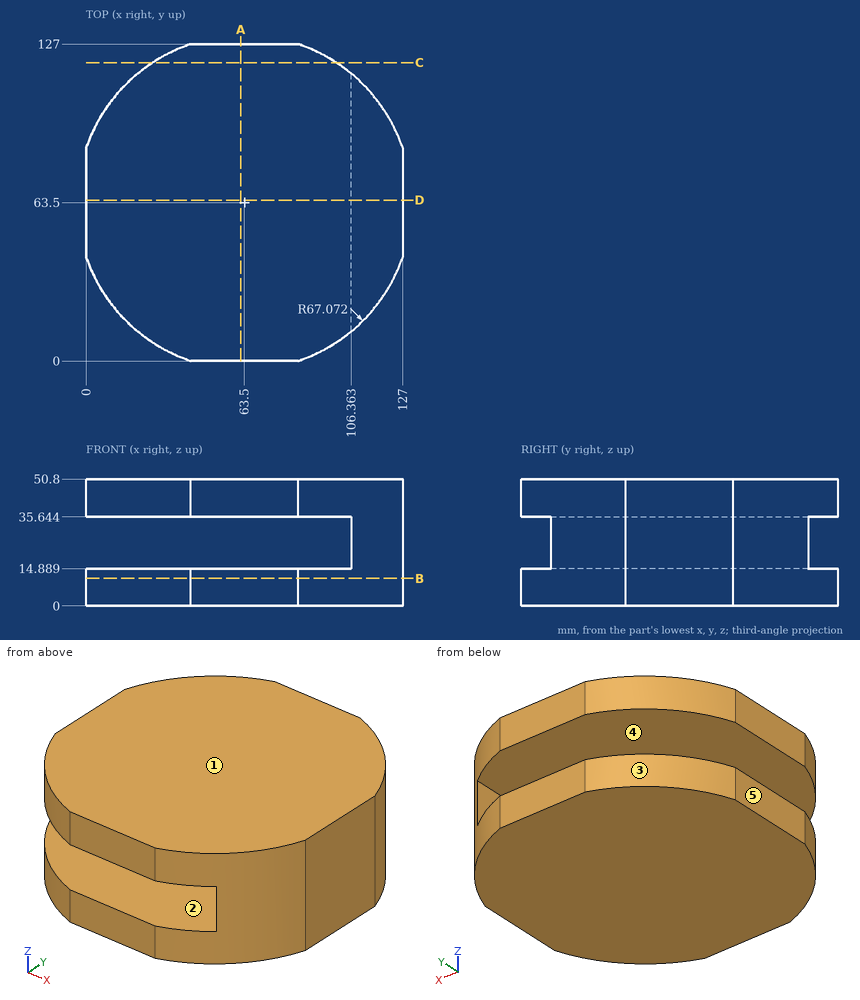
Study the drawing (mm; zero at the part's minimum x, y, z) and answer. A direction names the side the tool comes from. Give positions to 0.01 mm unless a question says otherwise; leave off trailing zeros. Order: outer loops, then holes, each group sorted by start corner. A loop starts at its lowest first (then second) coordinate and runs counter-clockwise, first axis right, second up. Notation, with made-up numbers: (57, -24.75) -> (80, -24.75) arc R20 ccw to (80, 14.25) -> close; hole circle Ø11 at (-10.75, 29). An arc over 180 degrees is marked (long way). Put each result on its own line as item: value.
Item 1: A cutting plane is placed at B-B on z = 11. Give the vertices of the cut face in (x, y) (1 decimal), plus the area to 3 significant figures.
Established:
outline: (0, 41.9) arc R67.1 ccw to (41.9, 0) -> (85.1, 0) arc R67.1 ccw to (127, 41.9) -> (127, 85.1) arc R67.1 ccw to (85.1, 127) -> (41.9, 127) arc R67.1 ccw to (0, 85.1) -> close
area: 13,700 mm^2
Item 2: For the marked faces 4 and 5, determine the directions among +Z, -Z, +X, -X, +Y, -Y from which every point of the face is accessible in a straight line to the end or side of a thin tool.
Established:
face 4: -X, +Y, -Y
face 5: +Z, -Z, -X, +Y, -Y
Item 3: Given P1, Ø1, axis at y = 95, z = 36, coming from the +X side; P2, Ø1.5, axis at x = 37.5, z = 34.5, coming from the -Y side; P3, Ø2, axis at y = 28, z = 29.5, coming from the -X side; P4, Ø10, axis at y = 20.5, z = 12.5, coming from the +X side, each flat-ended and moving along its own axis, determine where each tip first touches the part or whether it passes through.
Established:
P1: stops at x = 122.98
P2: passes through
P3: stops at x = 106.36
P4: stops at x = 118.77
Item 4: A cutting plane is placed at A-A on x = 62. Give the vertices of the cut face in (y, z).
Established:
outline: (0, 0) -> (127, 0) -> (127, 14.89) -> (0, 14.89) -> close; (0, 35.64) -> (127, 35.64) -> (127, 50.8) -> (0, 50.8) -> close
Item 5: For a pull along Z with two mould halves and no side action, classify the marked faces 1, 2 and 3 as released by +Z, released by -Z, zero draft, split by the parting line, or undercut.
Established:
face 1: released by +Z
face 2: undercut
face 3: zero draft
Item 6: Straight lines are drawn through the part: line 1 (Z direction, x = 36.5, y = 66.5); line 2 (X direction, y = 56, z = 20); line 3 (X direction, y = 120, z = 10) (1 decimal). For each, find the intervals that lie inside material, in ascending order.
Established:
line 1: z = 0 to 14.89, 35.64 to 50.8
line 2: x = 106.36 to 127
line 3: x = 27.4 to 99.6
Item 7: A cutting plane is placed at D-D on y = 64.5. Give the vertices of the cut face in (x, z), plus the area to 3 significant figures.
Established:
outline: (0, 0) -> (127, 0) -> (127, 50.8) -> (0, 50.8) -> (0, 35.64) -> (106.36, 35.64) -> (106.36, 14.89) -> (0, 14.89) -> close
area: 4,240 mm^2
Item 8: A cutting plane is placed at C-C on y = 119.5. Give the vertices of the cut face in (x, z).
Established:
outline: (26.59, 0) -> (100.41, 0) -> (100.41, 14.89) -> (26.59, 14.89) -> close; (26.59, 35.64) -> (100.41, 35.64) -> (100.41, 50.8) -> (26.59, 50.8) -> close
